Answer from the drawing. Dimensions are ordinates in mm from the lowest x, y and z of the part. A direction names the side the tool comes from. Give positions to 0.01 mm unless a question says otherwise; leave off trailing zeros. Write each loop counter-clockwise with the first axis right and the second up, starting at its lowest first coordinate (ties: lowest second). Pieces come first, ordered by that corner, then holes. Notation, with made-up numbers: (51, 41.5) -> (86, 41.5) arc R20 cw to (86, 75.5) -> close; hole circle Ø8 at (22, 11.25). An arc over 180 degrees is marked (long way). Write item = value, one per line.
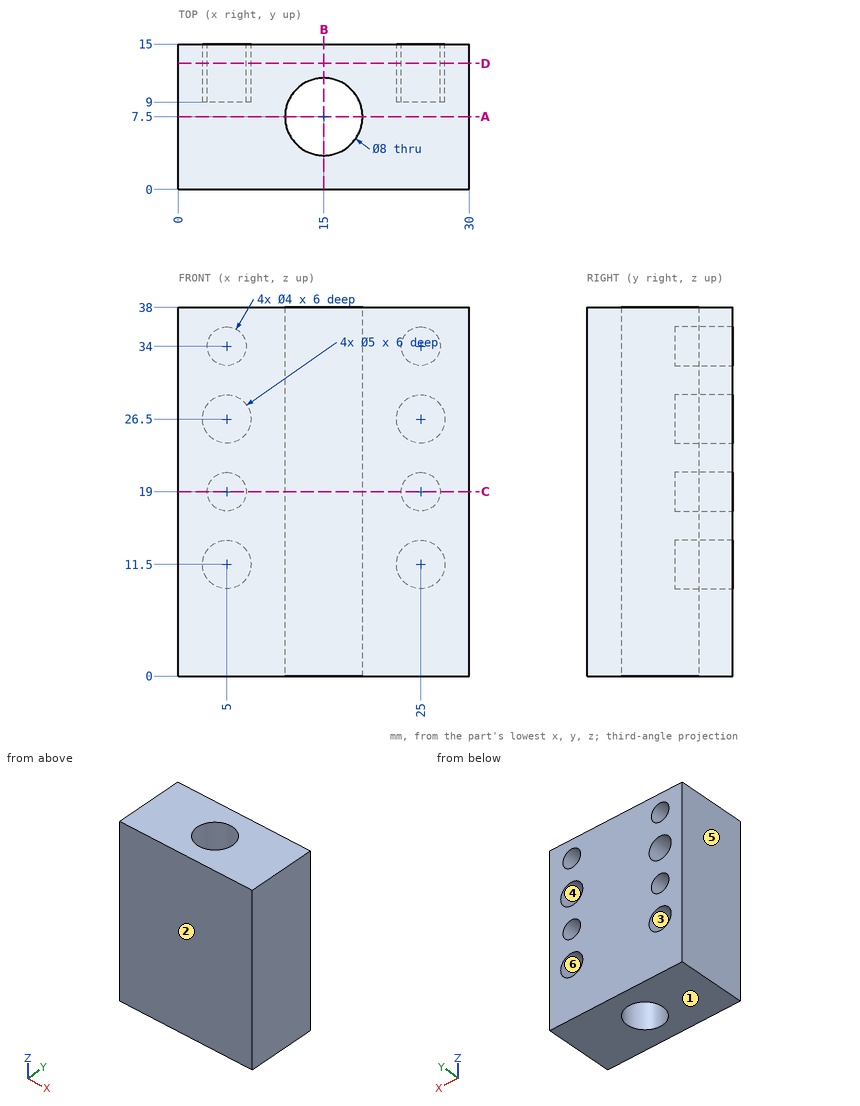
(1) The part is cut by section A-A on y = 7.5. Determine the outline of the cut face in (x, z), plus the area to 3 significant figures.
Checks:
outline = (0, 0) -> (11, 0) -> (11, 38) -> (0, 38) -> close; (19, 0) -> (30, 0) -> (30, 38) -> (19, 38) -> close
area = 836 mm²
(2) For a pull along Z with two mould halves and no side action, classify the marked faces 1, 2, 3 and 4 as released by +Z, released by -Z, zero draft, split by the parting line, or undercut.
Checks:
face_1 = released by -Z
face_2 = zero draft
face_3 = undercut
face_4 = undercut
(3) Given P1, Ø1.5, axis at x = 4, z = 11, coming from the +Y side, flat-ended and moving along its own axis, determine where the tip first touches the part or whether it passes through.
Checks:
P1 = 9
(4) The part is cut by section D-D on y = 13. Count the separate pieces of the cut face and the enclosed holes in it, plus the area to 3 significant figures.
Checks:
separate_pieces = 1
enclosed_holes = 8
area = 1,010 mm²
(5) The part is cut by section B-B on x = 15. Determine the outline of the cut face in (y, z).
Checks:
outline = (0, 0) -> (3.5, 0) -> (3.5, 38) -> (0, 38) -> close; (11.5, 0) -> (15, 0) -> (15, 38) -> (11.5, 38) -> close
(6) A tool of negligible diameter and unlimited length cuts with its end or side. For the marked faces 5 and 6, from which of +Z, -Z, +X, -X, +Y, -Y can it reach the whole face along a straight path? Write none if from no direction.
Checks:
face_5 = +Z, -Z, -X, +Y, -Y
face_6 = +Y
(7) Consider L1, parallel to X at y = 13.65, z = 26.5; L2, parallel to X at y = 12.65, z = 34; L3, parallel to Z at x = 25.75, y = 13. Determine where each line is inside the solid, lowest interval first.
Checks:
L1 = 0 to 2.5, 7.5 to 22.5, 27.5 to 30
L2 = 0 to 3, 7 to 23, 27 to 30
L3 = 0 to 9.12, 13.88 to 17.15, 20.85 to 24.12, 28.88 to 32.15, 35.85 to 38
(8) The part is cut by section C-C on z = 19. Determine the outline of the cut face in (x, y), plus the area to 3 significant figures.
Checks:
outline = (0, 0) -> (30, 0) -> (30, 15) -> (27, 15) -> (27, 9) -> (23, 9) -> (23, 15) -> (7, 15) -> (7, 9) -> (3, 9) -> (3, 15) -> (0, 15) -> close; hole circle Ø8 at (15, 7.5)
area = 352 mm²
